```python
from build123d import *

# Parameters (mm, degrees)
SKETCH_1_R      = 10
SKETCH_1_R_2    = 4
SKETCH_1_R_3    = 1.5
SKETCH_1_R_4    = 2
SKETCH_1_W      = 5.05
SKETCH_1_H      = 2.05
EXTRUDE_1_DEPTH = 2


with BuildPart() as part:
    # 草图1 → 凸台-拉伸1 (new body)
    with BuildSketch(Plane.XY):
        Polygon((317.453360513, 257.462931603), (317.453360513, 258.962931602), (314.853360513, 258.962931602), (314.853360513, 257.462931603), (311.853360513, 257.462931603), (311.853360513, 254.462931603), (314.853360513, 254.462931603), (314.853360513, 252.962931603), (317.453360513, 252.962931603), (317.453360513, 254.462931603), (319.953360513, 254.462931603), (319.953360513, 239.462931603), (321.953360513, 239.462931603), (321.953360513, 234.462931603), (319.953360513, 234.462931603), (319.953360513, 229.462931603), (321.953360513, 229.462931603), (321.953360513, 224.462931603), (319.953360513, 224.462931603), (319.953360513, 219.440879401), (179.953360513, 219.440879401), (179.953360513, 224.462931603), (177.953360513, 224.462931603), (177.953360513, 229.462931603), (179.953360513, 229.462931603), (179.953360513, 234.462931603), (177.953360513, 234.462931603), (177.953360513, 239.462931603), (179.953360513, 239.462931603), (179.953360513, 254.462931603), (182.453360513, 254.462931603), (182.453360513, 252.962931603), (185.053360513, 252.962931603), (185.053360513, 254.462931603), (188.053360513, 254.462931603), (188.053360513, 257.462931603), (185.053360513, 257.462931603), (185.053360513, 258.962931602), (182.453360513, 258.962931602), (182.453360513, 257.462931603), (179.953360513, 257.462931603), (179.953360513, 294.462931603), (182.453360513, 294.462931603), (182.453360513, 292.962931603), (185.053360513, 292.962931603), (185.053360513, 294.462931603), (188.053360513, 294.462931603), (188.053360513, 297.462931603), (185.053360513, 297.462931603), (185.053360513, 298.962931603), (182.453360513, 298.962931603), (182.453360513, 297.462931603), (179.953360513, 297.462931603), (179.953360513, 312.462931603), (177.953360513, 312.462931603), (177.953360513, 317.462931603), (179.953360513, 317.462931603), (179.953360513, 322.462931603), (177.953360513, 322.462931603), (177.953360513, 327.462931603), (179.953360513, 327.462931603), (179.953360513, 338.472931603), (317.453360513, 338.472931603), (319.953360513, 338.472931603), (319.953360513, 330.982931603), (319.953360513, 327.462931603), (321.953360513, 327.462931603), (321.953360513, 322.462931603), (319.953360513, 322.462931603), (319.953360513, 317.462931603), (321.953360513, 317.462931603), (321.953360513, 312.462931603), (319.953360513, 312.462931603), (319.953360513, 297.462931603), (317.453360513, 297.462931603), (317.453360513, 298.962931603), (314.853360513, 298.962931603), (314.853360513, 297.462931603), (311.853360513, 297.462931603), (311.853360513, 294.462931603), (314.853360513, 294.462931603), (314.853360513, 292.962931603), (317.453360513, 292.962931603), (317.453360513, 294.462931603), (319.953360513, 294.462931603), (319.953360513, 257.462931603), align=None)
        with Locations((249.953360513, 275.962931603)):
            Circle(SKETCH_1_R, mode=Mode.SUBTRACT)
        with Locations((249.953360513, 255.962931603)):
            Circle(SKETCH_1_R_2, mode=Mode.SUBTRACT)
        with Locations((229.953360513, 335.462931603)):
            Circle(SKETCH_1_R_3, mode=Mode.SUBTRACT)
        with Locations((269.953360513, 335.462931603)):
            Circle(SKETCH_1_R_3, mode=Mode.SUBTRACT)
        with Locations((229.953360513, 255.962931603)):
            Circle(SKETCH_1_R_4, mode=Mode.SUBTRACT)
        with Locations((229.953360513, 295.962931603)):
            Circle(SKETCH_1_R_4, mode=Mode.SUBTRACT)
        with Locations((269.953360513, 295.962931603)):
            Circle(SKETCH_1_R_4, mode=Mode.SUBTRACT)
        with Locations((269.953360513, 255.962931603)):
            Circle(SKETCH_1_R_4, mode=Mode.SUBTRACT)
        with Locations((288.953360513, 335.462931603)):
            Rectangle(SKETCH_1_W, SKETCH_1_H, mode=Mode.SUBTRACT)
        with Locations((298.953360513, 335.462931603)):
            Rectangle(SKETCH_1_W, SKETCH_1_H, mode=Mode.SUBTRACT)
        with Locations((200.953360513, 335.462931603)):
            Rectangle(SKETCH_1_W, SKETCH_1_H, mode=Mode.SUBTRACT)
        with Locations((210.953360513, 335.462931603)):
            Rectangle(SKETCH_1_W, SKETCH_1_H, mode=Mode.SUBTRACT)
    extrude(amount=EXTRUDE_1_DEPTH)


solid = part.part
```
Source: CAD feature listing. Evaluate the final solid. Frame: model axes, mm. Round coordinates to 2 decimals unless told otherwise and drop trailing zeros. Loops run counter-clockwise (first coordinate to the right, second up) from the corner with the lowest first, then second, coordinate; pieces in that order, holes last. Notation, with made-up numbers: M 57.5,67.5 L 95.5,67.5 A22 cw 95.5,97.5 Z; hole C -10.75,47.5 d10. An arc over 180 degrees is marked long. Use a Markdown table: item, result. Add a question column.
1. Line query: line 1 (Y direction, x = 201, z = 1.65); line 2 (X direction, y = 258.5, z = 1.85); line 3 (Y direction, x = 253, z = 0.65). Output: solid intervals per line, ascending.
2. Contact query for flat-ended pins moving along their axis: P1, Ø0.6, axis at y = 335, z = 0.5, coming from the +X side; P2, Ø0.8, axis at y = 254, z = 1, coming from the -X side; P3, Ø0.6, axis at x = 178.5, z = 1, coming from the +Y side; P4, Ø3.5, axis at x = 269.95, y = 255.96, coming from the +Z side. Output: stop coordinate, or through.
3. Section query D-D on z = 0.4. Give the number of separate pieces and of enclosed holes in the cut face, then the cut area to 3 significant figures.
4. Section query B-B on y = 272.5. Return the cut outline in (x, z).
5. Section query C-C on y = 310. Return the cut outline in (x, z).
6. Section query A-A on x = 298.5. Return the cut outline in (y, z).
7. Mould query, pull axis X, two halves, no side actions, for faces 1 (the cylindrical face through (231.861, 256.564, 0.986)), 2 (the flat face through (251, 293, 2)). Classes: pulls with the +X half, pulls with the -X half, needs draft (parallel to the pull), parting line crosses it, or undercut.
Reported:
| question | item | result |
|---|---|---|
| 1 | line 1 | y = 219.44 to 334.44, 336.49 to 338.47 |
| 1 | line 2 | x = 179.95 to 182.45, 185.05 to 246.86, 253.05 to 314.85, 317.45 to 319.95 |
| 1 | line 3 | y = 219.44 to 253.37, 258.55 to 266.44, 285.49 to 338.47 |
| 2 | P1 | stops at x = 319.95 |
| 2 | P2 | stops at x = 179.95 |
| 2 | P3 | stops at y = 327.46 |
| 2 | P4 | passes through |
| 3 | separate pieces | 1 |
| 3 | enclosed holes | 12 |
| 3 | area | 16,100 mm² |
| 4 | outline | M 179.95,0 L 240.57,0 L 240.57,2 L 179.95,2 Z; M 259.33,0 L 319.95,0 L 319.95,2 L 259.33,2 Z |
| 5 | outline | M 179.95,0 L 319.95,0 L 319.95,2 L 179.95,2 Z |
| 6 | outline | M 219.44,0 L 334.44,0 L 334.44,2 L 219.44,2 Z; M 336.49,0 L 338.47,0 L 338.47,2 L 336.49,2 Z |
| 7 | face 1 | undercut |
| 7 | face 2 | needs draft |
